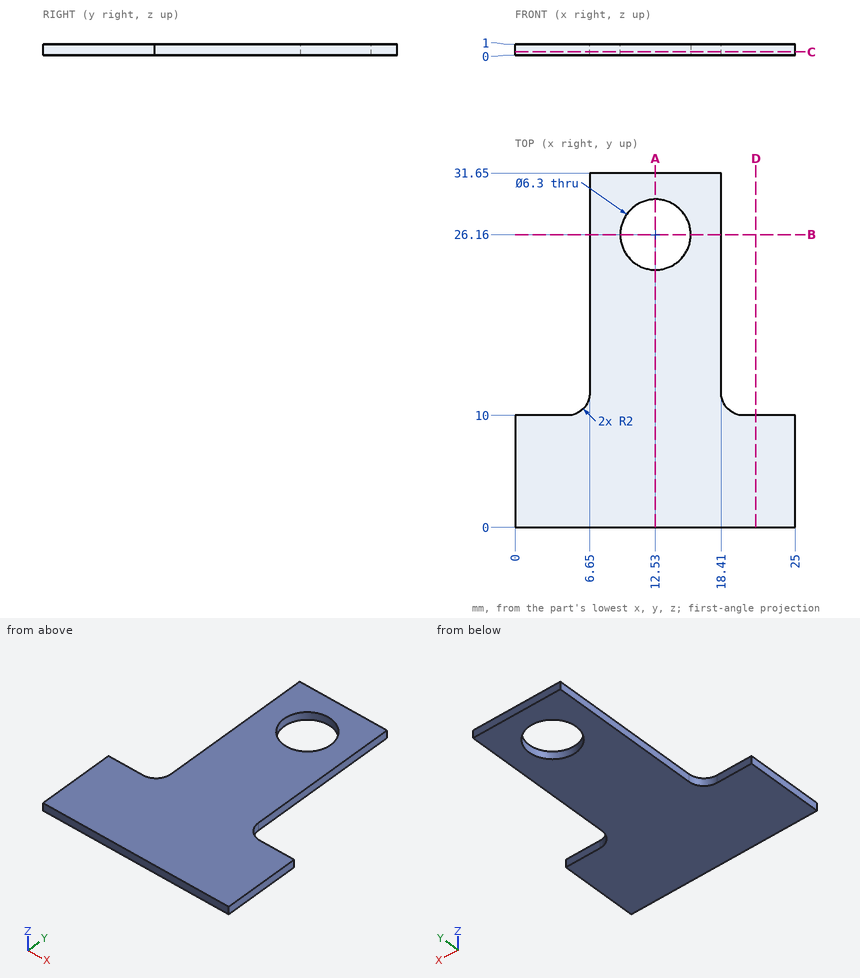
Drawing for the job (mm, zero at the part's lowest x, y, z). Coordinates: 2 decimals unless noted, no trailing zeros. Loops run counter-clockwise (first coordinate to the right, second up) from the corner with the lowest first, then second, coordinate; pieces in that order, holes last. Notation, with made-up numbers: (2.5, -13) - (52.5, -13) arc R24 ccw to (52.5, 20) - close; hole circle Ø2 at (55.25, 45.5). An arc over 180 degrees is marked (long way). Return JSON: item names as keys, results as strings.
1. Band-saw the part on A-A (x = 12.53). Give the cut face in (y, z).
Result:
{"outline": "(0, 0) - (23.01, 0) - (23.01, 1) - (0, 1) - close; (29.31, 0) - (31.65, 0) - (31.65, 1) - (29.31, 1) - close"}
2. Band-saw the part on C-C (z = 0.3). Give the cut face in (x, y), and give its area (3 significant figures).
Result:
{"outline": "(0, 0) - (25, 0) - (25, 10) - (20.41, 10) arc R2 cw to (18.41, 12) - (18.41, 31.65) - (6.65, 31.65) - (6.65, 12) arc R2 cw to (4.65, 10) - (0, 10) - close; hole circle Ø6.3 at (12.53, 26.16)", "area": "475 mm2"}
3. Band-saw the part on B-B (y = 26.16). Give the cut face in (x, z).
Result:
{"outline": "(6.65, 0) - (9.38, 0) - (9.38, 1) - (6.65, 1) - close; (15.68, 0) - (18.41, 0) - (18.41, 1) - (15.68, 1) - close"}
4. Probe L1, parallel to Y at x = 12.53, z = 0.55; L2, parallel to Y at x = 4, z = 0.8; L3, parallel to X at y = 15.5, z = 0.1. List the from-to ranges inside material, lowest first. Write a range as from..to.
Result:
{"L1": "y = 0..23.01, 29.31..31.65", "L2": "y = 0..10", "L3": "x = 6.65..18.41"}
5. Drop flat-ended pins along their axis: pin 1 (0.5 mm diameter, centred on x = 2.5, z = 0.5, fed in from +Y); pin 2 (0.5 mm diameter, centred on y = 18.5, z = 0.5, fed in from +X). Give the stop position or say it passes through.
Result:
{"pin 1": "stops at y = 10", "pin 2": "stops at x = 18.41"}
6. Band-saw the part on D-D (x = 21.5). Give the cut face in (y, z).
Result:
{"outline": "(0, 0) - (10, 0) - (10, 1) - (0, 1) - close"}
